The listing builds one solid part. Answer for the finished solid, in the listing's coordinates (mm). A direction names the side the tool comes from. Coordinates: 2 decimals unless noted, no trailing zeros. Write each loop counter-clockwise with the first axis right and the second up, starting at its lowest first coordinate (ties: lowest second). Pieces come first, ordered by that corner, then holes.
from build123d import *

# Parameters (mm, degrees)
SKETCH1_W                = 39
SKETCH1_H                = 7.38
BOSS_EXTRUDE1_DEPTH      = 7.76
SKETCH2_R                = 2.4
CUT_EXTRUDE1_DEPTH       = 7.76
CUT_EXTRUDE2_OUTLINE_R   = 3.1
CUT_EXTRUDE2_OUTLINE_R_2 = 2.4
CUT_EXTRUDE2_DEPTH       = 0.8
CUT_EXTRUDE3_START       = 6.96
CUT_EXTRUDE3_OUTLINE_R   = 3.1
CUT_EXTRUDE3_OUTLINE_R_2 = 2.4
CUT_EXTRUDE3_DEPTH       = 0.8
LPATTERN3_COUNT          = 3
LPATTERN3_PITCH          = 7.79
LPATTERN6_COUNT          = 3
LPATTERN6_PITCH          = 7.79
FILLET1_R                = 3.69
FILLET2_R                = 3.69
FILLET3_R                = 3.69
FILLET4_R                = 3.69
SKETCH3_R                = 3.1
BOSS_EXTRUDE2_DEPTH      = 7.76
BOSS_EXTRUDE3_START      = -7.76
SKETCH4_R                = 3.1
BOSS_EXTRUDE3_DEPTH      = 7.76
SKETCH6_R                = 1.6
BOSS_EXTRUDE4_DEPTH      = 7.5
SKETCH10_R               = 1.6
BOSS_EXTRUDE5_DEPTH      = 8


# Read off the part's stored shape, not the designer's step: Cut-Extrude2, Cut-Extrude3
with BuildPart() as part:
    # Sketch1 → Boss-Extrude1 (new body)
    with BuildSketch(Plane.XY):
        with Locations((19.5, 3.69)):
            Rectangle(SKETCH1_W, SKETCH1_H)
    extrude(amount=BOSS_EXTRUDE1_DEPTH)

    # Sketch2 → Cut-Extrude1 (cut)
    with BuildSketch(Plane.XY.offset(7.76)):
        with Locations((19.5, 3.69)):
            Circle(SKETCH2_R)
    cut_extrude1 = extrude(amount=-CUT_EXTRUDE1_DEPTH, mode=Mode.SUBTRACT)

    # Cut-Extrude2 outline → Cut-Extrude2 (cut)
    with BuildSketch(Plane.XY):
        with Locations((19.5, 3.69)):
            Circle(CUT_EXTRUDE2_OUTLINE_R)
        with Locations((19.5, 3.69)):
            Circle(CUT_EXTRUDE2_OUTLINE_R_2, mode=Mode.SUBTRACT)
    cut_extrude2 = extrude(amount=CUT_EXTRUDE2_DEPTH, mode=Mode.SUBTRACT)

    # Cut-Extrude3 outline → Cut-Extrude3 (cut)
    with BuildSketch(Plane.XY.offset(CUT_EXTRUDE3_START)):
        with Locations((19.5, 3.69)):
            Circle(CUT_EXTRUDE3_OUTLINE_R)
        with Locations((19.5, 3.69)):
            Circle(CUT_EXTRUDE3_OUTLINE_R_2, mode=Mode.SUBTRACT)
    cut_extrude3 = extrude(amount=CUT_EXTRUDE3_DEPTH, mode=Mode.SUBTRACT)

    # LPattern3: Cut-Extrude1, Cut-Extrude2, Cut-Extrude3 ×3
    with Locations(*[(-i * LPATTERN3_PITCH, 0, 0) for i in range(1, LPATTERN3_COUNT)]):
        add(cut_extrude1, mode=Mode.SUBTRACT)
        add(cut_extrude2, mode=Mode.SUBTRACT)
        add(cut_extrude3, mode=Mode.SUBTRACT)

    # LPattern6: Cut-Extrude1, Cut-Extrude2, Cut-Extrude3 ×3
    with Locations(*[(i * LPATTERN6_PITCH, 0, 0) for i in range(1, LPATTERN6_COUNT)]):
        add(cut_extrude1, mode=Mode.SUBTRACT)
        add(cut_extrude2, mode=Mode.SUBTRACT)
        add(cut_extrude3, mode=Mode.SUBTRACT)

    # Fillet1
    fillet1_edges = [part.edges().sort_by_distance(p)[0] for p in [
        (0, 7.38, 3.88),
    ]]
    fillet(fillet1_edges, radius=FILLET1_R)

    # Fillet2
    fillet2_edges = [part.edges().sort_by_distance(p)[0] for p in [
        (0, 0, 3.88),
    ]]
    fillet(fillet2_edges, radius=FILLET2_R - 0.0001)  # a hair under: the kernel refuses the full size

    # Fillet3
    fillet3_edges = [part.edges().sort_by_distance(p)[0] for p in [
        (39, 7.38, 3.88),
    ]]
    fillet(fillet3_edges, radius=FILLET3_R)

    # Fillet4
    fillet4_edges = [part.edges().sort_by_distance(p)[0] for p in [
        (39, 0, 3.88),
    ]]
    fillet(fillet4_edges, radius=FILLET4_R - 0.0001)  # a hair under: the kernel refuses the full size

    # Sketch3 → Boss-Extrude2 (add)
    with BuildSketch(Plane(origin=(0, 0, 0), x_dir=(-1, 0, 0), z_dir=(0, 0, -1))):
        with Locations((-35.08, 3.69)):
            Circle(SKETCH3_R)
    extrude(amount=-BOSS_EXTRUDE2_DEPTH)

    # Sketch4 → Boss-Extrude3 (add)
    with BuildSketch(Plane.XY.offset(7.76).offset(BOSS_EXTRUDE3_START)):
        with Locations((3.92, 3.69)):
            Circle(SKETCH4_R)
    extrude(amount=BOSS_EXTRUDE3_DEPTH)

    # Sketch6 → Boss-Extrude4 (add)
    with BuildSketch(Plane.XY.offset(7.76)):
        with Locations(Location((1, 3.69, 0), (0, 0, 243.655122674))):
            Circle(SKETCH6_R)
        with Locations(Location((38, 3.69, 0), (0, 0, 296.344877326))):
            Circle(SKETCH6_R)
    extrude(amount=BOSS_EXTRUDE4_DEPTH)

    # Sketch10 → Boss-Extrude5 (add)
    with BuildSketch(Plane(origin=(0, 0, 0), x_dir=(-1, 0, 0), z_dir=(0, 0, -1))):
        with Locations(Location((-38, 3.69, 0), (0, 0, 116.344877326))):
            Circle(SKETCH10_R)
        with Locations(Location((-1, 3.69, 0), (0, 0, 63.655122674))):
            Circle(SKETCH10_R)
    extrude(amount=-BOSS_EXTRUDE5_DEPTH)


solid = part.part
Q1. Find the intervals of material crossed by probe 1 along Y at (x, z) = (27.29, 5); probe 2 along Y at (x, z) = (27.29, 0.6); probe 3 along X at (y, z) = (3, 3.75), in increasing order.
Answers below:
probe 1: y = 0 to 1.29, 6.09 to 7.38
probe 2: y = 0 to 0.59, 6.79 to 7.38
probe 3: x = -0.44 to 9.41, 14.01 to 17.2, 21.8 to 24.99, 29.59 to 39.44
Q2. The part is cut by section C-C, the plane z = 14. Write down the section's boundary in (x, y).
Answers below:
outline: circle Ø3.2 at (1, 3.69); circle Ø3.2 at (38, 3.69)
Q3. Determine the mould class of faces 1 (the face through (37.375, 0.632, 3.934)), 2 (the face through (9.25, 1.804, 0.394)), 3 (the face through (1, 4, 15.26)) for opening direction X: released by +X, released by -X, zero draft, split by the parting line, or undercut.
Answers below:
face 1: released by +X
face 2: undercut
face 3: zero draft
Q4. The part is cut by section A-A, the plane x = 27.29. Write down the section's boundary in (y, z).
Answers below:
outline: (0, 0) - (0.59, 0) - (0.59, 0.8) - (1.29, 0.8) - (1.29, 6.96) - (0.59, 6.96) - (0.59, 7.76) - (0, 7.76) - close; (6.09, 0.8) - (6.79, 0.8) - (6.79, 0) - (7.38, 0) - (7.38, 7.76) - (6.79, 7.76) - (6.79, 6.96) - (6.09, 6.96) - close
Q5. Which of the six approach directions +Z, -Z, +X, -X, +Y, -Y give full straight-line access (tool end or side, diameter ignored) to faces 4 (the face through (24.892, 3.796, 3.923)), 5 (the face through (9, 3, 0.8)), 6 (the face through (17.04, 1.804, 7.354))?
Answers below:
face 4: +Z, -Z
face 5: -Z
face 6: +Z
Q6. Given pin 1 (3.5 mm diameter, centred on x = 13.5, y = 2, fed in from +Z); pin 2 (1.5 mm diameter, centred on y = 5, z = 10.5, fed in from -X); pin 3 (1.9 mm diameter, centred on x = 12, y = 4.5, fed in from -Z) (1 decimal); pin 4 (4 mm diameter, centred on y = 1, z = 3.5, fed in from -X), each flat-ended and moving along its own axis, determine where each tip first touches the part or whether it passes through.
Answers below:
pin 1: stops at z = 7.76
pin 2: stops at x = -0.5
pin 3: passes through
pin 4: stops at x = -0.44
Q7. The part is cut by section B-B, the plane z = 1.5. Write down the section's boundary in (x, y), then the cut area to 3 significant figures.
Answers below:
outline: (0.29, 2.26) arc R3.69 ccw to (3.69, 0) - (35.31, 0) arc R3.69 ccw to (38.71, 2.26) arc R1.6 ccw to (38.71, 5.12) arc R3.69 ccw to (35.31, 7.38) - (3.69, 7.38) arc R3.69 ccw to (0.29, 5.12) arc R1.6 ccw to start; hole circle Ø4.8 at (11.71, 3.69); hole circle Ø4.8 at (19.5, 3.69); hole circle Ø4.8 at (27.29, 3.69)
area: 224 mm2
Q8. The part is cut by section D-D, the plane x = 38. Write down the section's boundary in (y, z), then the cut area to 3 significant figures.
Answers below:
outline: (1.16, 0) - (6.22, 0) - (6.22, 7.76) - (5.29, 7.76) - (5.29, 15.26) - (2.09, 15.26) - (2.09, 7.76) - (1.16, 7.76) - close
area: 63.2 mm2
